The model under review builds one solid part; all positions refer to its coordinate system, in mm. Face numbers are marked on the shaded views. A direction names the side the tool comes from. Coordinates: 2 decimals unless noted, no trailing zeros. Loops run counter-clockwise (first coordinate to the right, second up) from the corner with the lowest first, then second, coordinate; pieces in that order, holes last. Notation, with made-up numbers: M 25,-20.5 L 73,-20.5 A21 cw 73,-14.5 Z; hole C -30,-28.75 d4. An arc over 180 degrees is marked long. One line per item, written item: value.
```python
from build123d import *

# Parameters (mm, degrees)
SKETCH1_R           = 14
BOSS_EXTRUDE1_DEPTH = 7
SKETCH2_R           = 25
SKETCH2_R_2         = 14
BOSS_EXTRUDE2_DEPTH = 7.5


with BuildPart() as part:
    # Sketch1 → Boss-Extrude1 (new body, symmetric)
    with BuildSketch(Plane.XY):
        with BuildLine():
            Line((-19.5, 35), (19.5, 35))
            ThreePointArc((19.5, 35), (28.332479027, 28.332479027), (35, 19.5))
            Line((35, 19.5), (35, -19.5))
            ThreePointArc((35, -19.5), (28.332479027, -28.332479027), (19.5, -35))
            Line((19.5, -35), (-19.5, -35))
            ThreePointArc((-19.5, -35), (-28.332479027, -28.332479027), (-35, -19.5))
            Line((-35, -19.5), (-35, 19.5))
            ThreePointArc((-35, 19.5), (-28.332479027, 28.332479027), (-19.5, 35))
        make_face()
        with Locations((-0.04820778, -0.04820778)):
            Circle(SKETCH1_R, mode=Mode.SUBTRACT)
    extrude(amount=BOSS_EXTRUDE1_DEPTH, both=True)

    # Sketch2 → Boss-Extrude2 (add, symmetric)
    with BuildSketch(Plane.XY):
        Circle(SKETCH2_R)
        Circle(SKETCH2_R_2, mode=Mode.SUBTRACT)
    extrude(amount=BOSS_EXTRUDE2_DEPTH, both=True)


solid = part.part
```
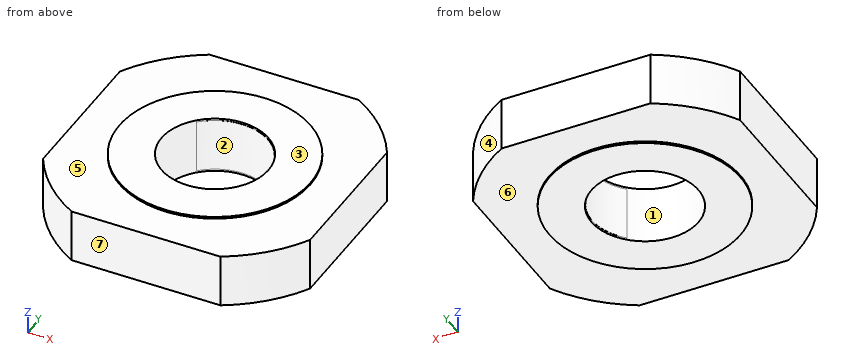
(1) Add section C-C on z = -3. State the section outline as (x, y) points, then the cut area to 3 significant figures.
Checks:
outline: M -35,-19.5 A40 ccw -19.5,-35 L 19.5,-35 A40 ccw 35,-19.5 L 35,19.5 A40 ccw 19.5,35 L -19.5,35 A40 ccw -35,19.5 Z; hole M -9.92,9.88 A14 ccw 9.88,-9.92 A14 ccw Z
area: 3,900 mm^2
(2) Insertion check: pin 1 Ø12 at (x, y) = (-3, 7) entering from -Z; pin 2 Ø4 at (x, z) = (24, 1) entering from -Y; pin 3 Ø1 at (x, z) = (-23, -3) entering from -Y. Each pin has a flat end and moves straight along its axis. Give the tip position at first contact, or say it passes through.
Checks:
pin 1: through
pin 2: y = -33.49
pin 3: y = -33.15
(3) Add section D-D on y = -23.5. State the section outline as (x, z) points.
Checks:
outline: M -32.45,-7 L -8.53,-7 L -8.53,-7.5 L 8.53,-7.5 L 8.53,-7 L 32.45,-7 L 32.45,7 L 8.53,7 L 8.53,7.5 L -8.53,7.5 L -8.53,7 L -32.45,7 Z
(4) Draft analysis for pull direction Y (two halves, no side actions). For the marked faces 1, 2, 3 and 4, state which applies: pulls with the +Y half, pulls with the -Y half, needs draft (parallel to the pull), parting line crosses it, or undercut.
Checks:
face 1: undercut
face 2: undercut
face 3: needs draft
face 4: pulls with the +Y half
(5) Add section A-A on x = 0. State the section outline as (y, z) points.
Checks:
outline: M -35,-7 L -25,-7 L -25,-7.5 L -14,-7.5 L -14,7.5 L -25,7.5 L -25,7 L -35,7 Z; M 13.95,-7 L 14,-7 L 14,-7.5 L 25,-7.5 L 25,-7 L 35,-7 L 35,7 L 25,7 L 25,7.5 L 14,7.5 L 14,7 L 13.95,7 Z
(6) To check wall thickness, follow L1, parallel to Y at x = 0, z = 1.25; L2, parallel to Z at x = -22, y = 29; L3, parallel to X at y = 1, z = -4.75. State the ranges of each line that lie inside material, in increasing order. Write a range as [from, to].
Checks:
L1: [-35, -14], [13.95, 35]
L2: [-7, 7]
L3: [-35, -13.96], [13.91, 35]
(7) Tool access review of the marked faces 5, 6 and 7: name each direction out of +Z, -Z, +X, -X, +Y, -Y from which nothing blocks a thin tool from reaching the whole face with its end or side.
Checks:
face 5: +Z
face 6: -Z
face 7: +Z, -Z, +X, -X, -Y
